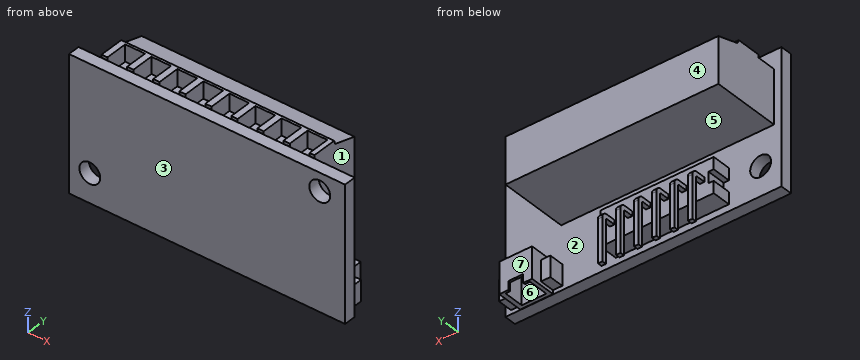
```python
from build123d import *

# Parameters (mm, degrees)
SKETCH1_W           = 37.1
SKETCH1_H           = 18.06
SKETCH1_R           = 1.4
BOSS_EXTRUDE1_DEPTH = 1.6
SKETCH2_W           = 0.7
SKETCH2_H           = 1.5
BOSS_EXTRUDE2_DEPTH = 2.54
SKETCH4_W           = 0.6
SKETCH4_H           = 0.6
LPATTERN1_COUNT     = 6
LPATTERN1_PITCH     = 2.42
SKETCH6_W           = 28.6
SKETCH6_H           = 7.6
BOSS_EXTRUDE3_DEPTH = 9.3
CUT_EXTRUDE1_REACH  = 38.1
SKETCH7_W           = 0.4
SKETCH7_H           = 2.6
SKETCH8_W           = 2.65
SKETCH8_H           = 5.571671588
CUT_EXTRUDE2_DEPTH  = 2.25
SKETCH9_W           = 4.4
SKETCH9_H           = 4.21
BOSS_EXTRUDE4_DEPTH = 3.5
SKETCH10_W          = 6.9
SKETCH10_H          = 2.792271398
BOSS_EXTRUDE5_DEPTH = 2
SKETCH11_W          = 3.3
SKETCH11_H          = 2.7
CUT_EXTRUDE3_DEPTH  = 3.5
CUT_EXTRUDE4_REACH  = 7.1
SKETCH12_W          = 1.985213288
SKETCH12_H          = 1.157017581


with BuildPart() as part:
    # Sketch1 → Boss-Extrude1 (new body)
    with BuildSketch(Plane(origin=(0, 0, 0), x_dir=(1, 0, 0), z_dir=(0, 1, 0))):
        with Locations((18.55, 9.03)):
            Rectangle(SKETCH1_W, SKETCH1_H)
        with Locations(Location((33.7, 2.4, 0), (0, 0, 270))):  # turned: the seam where the file's is
            Circle(SKETCH1_R, mode=Mode.SUBTRACT)
        with Locations(Location((2.8, 14.16, 0), (0, 0, 270))):  # turned: the seam where the file's is
            Circle(SKETCH1_R, mode=Mode.SUBTRACT)
    extrude(amount=BOSS_EXTRUDE1_DEPTH)

    # Sketch2 → Boss-Extrude2 (add)
    with BuildSketch(Plane(origin=(0, 1.6, 0), x_dir=(1, 0, 0), z_dir=(0, 1, 0))):
        Polygon((7.060184456, 17.16), (22.260184456, 17.16), (22.260184456, 15.56), (21.580184456, 15.56), (21.580184456, 14.06), (22.260184456, 14.06), (22.260184456, 12.46), (7.060184456, 12.46), (7.060184456, 14.06), (7.760184456, 14.06), (7.760184456, 15.56), (7.060184456, 15.56), align=None)
        with Locations((9.830184456, 14.81)):
            Rectangle(SKETCH2_W, SKETCH2_H, mode=Mode.SUBTRACT)
        with Locations((12.250184456, 14.81)):
            Rectangle(SKETCH2_W, SKETCH2_H, mode=Mode.SUBTRACT)
        with Locations((14.670184456, 14.81)):
            Rectangle(SKETCH2_W, SKETCH2_H, mode=Mode.SUBTRACT)
        with Locations((17.090184456, 14.81)):
            Rectangle(SKETCH2_W, SKETCH2_H, mode=Mode.SUBTRACT)
        with Locations((19.510184456, 14.81)):
            Rectangle(SKETCH2_W, SKETCH2_H, mode=Mode.SUBTRACT)
    extrude(amount=BOSS_EXTRUDE2_DEPTH)

    # Sweep1: sweep along a path in Sketch3
    with BuildLine(Plane.ZY.offset(-8.610184456)) as sweep1_path:
        Line((-14.533057121, 4.14), (-14.533057121, 5.39))
        ThreePointArc((-14.533057121, 5.39), (-14.752727035, 5.920330086), (-15.283057121, 6.14))
        Line((-15.283057121, 6.14), (-21.033057121, 6.14))
    # Sketch4 → Sweep1 (sweep)
    with BuildSketch(Plane(origin=(0, 4.14, 0), x_dir=(1, 0, 0), z_dir=(0, 1, 0))):
        with Locations((8.610184456, 14.833057121)):
            Rectangle(SKETCH4_W, SKETCH4_H)
    sweep1 = sweep(path=sweep1_path.line)

    # LPattern1: Sweep1 ×6
    with Locations(*[(i * LPATTERN1_PITCH, 0, 0) for i in range(1, LPATTERN1_COUNT)]):
        add(sweep1)

    # Sketch6 → Boss-Extrude3 (add)
    with BuildSketch(Plane(origin=(0, 1.6, 0), x_dir=(1, 0, 0), z_dir=(0, 1, 0))):
        with Locations((15.3, 5.8)):
            Rectangle(SKETCH6_W, SKETCH6_H)
    extrude(amount=BOSS_EXTRUDE3_DEPTH)

    # Sketch7 → Cut-Extrude1 (cut, up to next)
    with BuildSketch(Plane.ZY.offset(-1), mode=Mode.PRIVATE) as cut_extrude1_sk1:
        Polygon((-2, 7.5), (-2.508141267, 7.68870454), (-3.4, 10.9), (-2, 10.9), align=None)
    cut_extrude1_tool1 = extrude(cut_extrude1_sk1.sketch, amount=-CUT_EXTRUDE1_REACH, mode=Mode.PRIVATE) & part.part
    add(cut_extrude1_tool1.solids().sort_by_distance((1, 9.514948, -2.506498))[0], mode=Mode.SUBTRACT)
    # Sketch7 → Cut-Extrude1 (cut, up to next)
    with BuildSketch(Plane.ZY.offset(-1), mode=Mode.PRIVATE) as cut_extrude1_sk2:
        with Locations((-2.2, 2.9)):
            Rectangle(SKETCH7_W, SKETCH7_H)
    cut_extrude1_tool2 = extrude(cut_extrude1_sk2.sketch, amount=-CUT_EXTRUDE1_REACH, mode=Mode.PRIVATE) & part.part
    add(cut_extrude1_tool2.solids().sort_by_distance((1, 2.9, -2.2))[0], mode=Mode.SUBTRACT)

    # Sketch8 → Cut-Extrude2 (cut)
    with BuildSketch(Plane.XY.offset(-2)):
        with Locations((3.120484252, 4.385835794)):
            Rectangle(SKETCH8_W, SKETCH8_H)
        with Locations((6.620484252, 4.385835794)):
            Rectangle(SKETCH8_W, SKETCH8_H)
        with Locations((10.120484252, 4.385835794)):
            Rectangle(SKETCH8_W, SKETCH8_H)
        with Locations((13.620484252, 4.385835794)):
            Rectangle(SKETCH8_W, SKETCH8_H)
        with Locations((17.120484252, 4.385835794)):
            Rectangle(SKETCH8_W, SKETCH8_H)
        with Locations((20.620484252, 4.385835794)):
            Rectangle(SKETCH8_W, SKETCH8_H)
        with Locations((24.120484252, 4.385835794)):
            Rectangle(SKETCH8_W, SKETCH8_H)
        with Locations((27.620484252, 4.385835794)):
            Rectangle(SKETCH8_W, SKETCH8_H)
    extrude(amount=-CUT_EXTRUDE2_DEPTH, mode=Mode.SUBTRACT)

    # Sketch9 → Boss-Extrude4 (add)
    with BuildSketch(Plane(origin=(0, 1.6, 0), x_dir=(1, 0, 0), z_dir=(0, 1, 0))):
        with Locations((32.9, 15.905)):
            Rectangle(SKETCH9_W, SKETCH9_H)
    extrude(amount=BOSS_EXTRUDE4_DEPTH)

    # Sketch10 → Boss-Extrude5 (add)
    with BuildSketch(Plane(origin=(0, 1.6, 0), x_dir=(1, 0, 0), z_dir=(0, 1, 0))):
        with Locations((32.9, 16.113864301)):
            Rectangle(SKETCH10_W, SKETCH10_H)
    extrude(amount=BOSS_EXTRUDE5_DEPTH)

    # Sketch11 → Cut-Extrude3 (cut)
    with BuildSketch(Plane(origin=(0, 0, -18.01), x_dir=(-1, 0, 0), z_dir=(0, 0, -1))):
        with Locations((-32.852042443, 3.45)):
            Rectangle(SKETCH11_W, SKETCH11_H)
    extrude(amount=-CUT_EXTRUDE3_DEPTH, mode=Mode.SUBTRACT)

    # Sketch12 → Cut-Extrude4 (cut, up to next)
    with BuildSketch(Plane(origin=(0, 5.1, 0), x_dir=(1, 0, 0), z_dir=(0, 1, 0)), mode=Mode.PRIVATE) as cut_extrude4_sk1:
        with Locations((32.883783696, 17.43149121)):
            Rectangle(SKETCH12_W, SKETCH12_H)
    cut_extrude4_tool1 = extrude(cut_extrude4_sk1.sketch, amount=-CUT_EXTRUDE4_REACH, mode=Mode.PRIVATE) & part.part
    add(cut_extrude4_tool1.solids().sort_by_distance((32.883784, 5.1, -17.431491))[0], mode=Mode.SUBTRACT)


solid = part.part
```
Build history of the part. All positions in model axes, mm. Face numbers are marked on the shaded views. A direction names the side the tool comes from. Give positions to 0.01 mm unless a question says otherwise; leave off trailing zeros. Loops run counter-clockwise (first coordinate to the right, second up) from the corner with the lowest first, then second, coordinate; pieces in that order, holes last.
1) Drop flat-ended pins along their axis: P1, Ø0.5, axis at x = 18.5, y = 5, coming from the +Z side; P2, Ø3, axis at y = 5, z = -2.5, coming from the +X side; P3, Ø0.7, axis at x = 13.5, z = -17, coming from the +Y side. Give the stop position or say it passes through.
Values follow:
P1: stops at z = -2
P2: stops at x = 29.6
P3: stops at y = 6.14
2) Band-saw the part on A-A on x = 2.8. List the corners of the cut face in (y, z).
Values follow:
outline: (0, -18.06) - (1.6, -18.06) - (1.6, -15.56) - (0, -15.56) - close; (0, -12.76) - (1.6, -12.76) - (1.6, -9.6) - (10.9, -9.6) - (10.9, -3.4) - (7.69, -2.51) - (7.5, -2) - (7.17, -2) - (7.17, -4.25) - (1.6, -4.25) - (1.6, 0) - (0, 0) - close
3) Band-saw the part on B-B on z = -6.5. List the corners of the cut face in (x, y).
Values follow:
outline: (0, 0) - (37.1, 0) - (37.1, 1.6) - (29.6, 1.6) - (29.6, 10.9) - (1, 10.9) - (1, 1.6) - (0, 1.6) - close
4) Two-plate mould, pull along Y, no slides. Class the marked faces 1, 2, 3 and 4: released by +Y, released by -Y, zero draft, split by the parting line, or undercut.
Values follow:
face 1: zero draft
face 2: undercut
face 3: released by -Y
face 4: released by +Y
5) Probe line 1 along X through (y, z) = (5.25, -15); line 2 along Z through (x, y) = (11, 3); line 3 along X through (y, z) = (0.65, -14.16). List the from-to ranges inside material, lowest first.
Values follow:
line 1: x = 8.31 to 8.91, 10.73 to 11.33, 13.15 to 13.75, 15.57 to 16.17, 17.99 to 18.59, 20.41 to 21.01
line 2: z = -17.16 to -12.46, -9.6 to -4.25
line 3: x = 0 to 1.4, 4.2 to 37.1
6) Band-saw the part on C-C on y = 9. List the corners of the cut face in (x, z).
Values follow:
outline: (1, -9.6) - (29.6, -9.6) - (29.6, -2.87) - (1, -2.87) - close
7) 3-axis set-ups, long thin cutter, end or side, ignore diameter. For the marked faces 5, 6 and 7: which of +Z, -Z, +X, -X, +Y, -Y reach the whole face in a straight line?
Values follow:
face 5: +X, -X, +Y
face 6: -Z
face 7: +Z, -Z, +X, +Y
